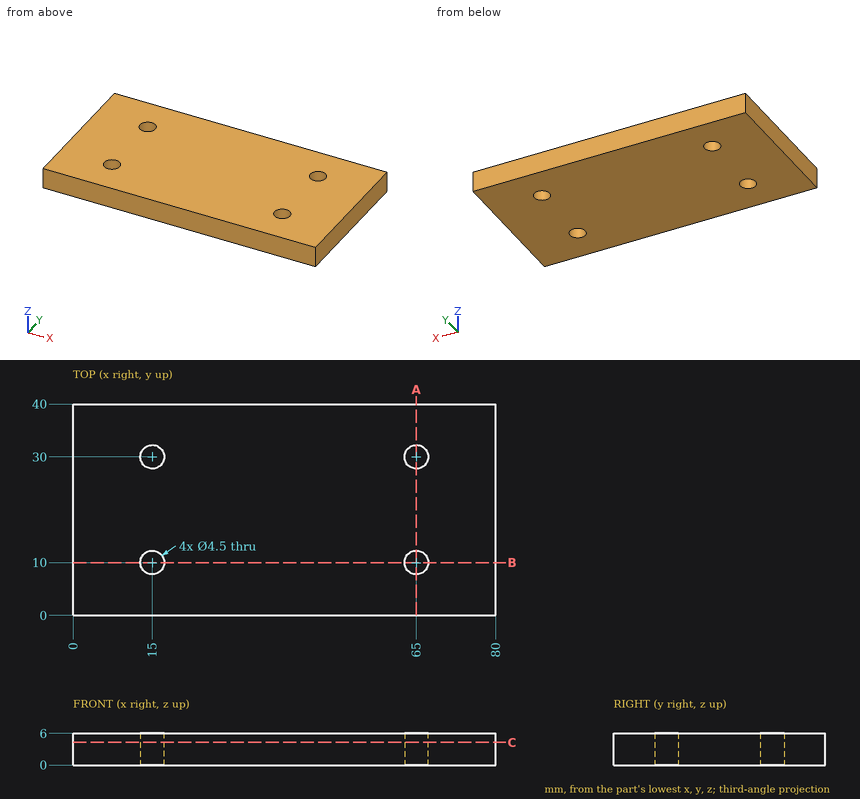
Drawing for the job (mm, zero at the part's lowest x, y, z). Coordinates: 2 decimals unless noted, no trailing zeros. Loops run counter-clockwise (first coordinate to the right, second up) from the corner with the lowest first, then second, coordinate; pieces in that order, holes last. Notation, with made-up numbers: (6, 50.5) - (51, 50.5) arc R14 cw to (51, 61.5) - close; hole circle Ø7 at (-10, 35.25). An arc over 180 degrees is marked (long way). Return JSON: item names as keys, results as strings.
1. Probe L1, parallel to Y at x = 65, z = 4; L2, parallel to X at y = 10, z = 3.65; L3, parallel to X at y = 29, z = 0.5. List the from-to ranges inside material, lowest first. Write a range as from..to.
Result:
{"L1": "y = 0..7.75, 12.25..27.75, 32.25..40", "L2": "x = 0..12.75, 17.25..62.75, 67.25..80", "L3": "x = 0..12.98, 17.02..62.98, 67.02..80"}
2. Band-saw the part on C-C (z = 4.3). Give the cut face in (x, y), and give its area (3 significant figures).
Result:
{"outline": "(0, 0) - (80, 0) - (80, 40) - (0, 40) - close; hole circle Ø4.5 at (15, 10); hole circle Ø4.5 at (15, 30); hole circle Ø4.5 at (65, 10); hole circle Ø4.5 at (65, 30)", "area": "3,140 mm2"}
3. Band-saw the part on B-B (y = 10). Give the cut face in (x, z), and give its area (3 significant figures).
Result:
{"outline": "(0, 0) - (12.75, 0) - (12.75, 6) - (0, 6) - close; (17.25, 0) - (62.75, 0) - (62.75, 6) - (17.25, 6) - close; (67.25, 0) - (80, 0) - (80, 6) - (67.25, 6) - close", "area": "426 mm2"}
4. Band-saw the part on A-A (x = 65). Give the cut face in (y, z), and give its area (3 significant figures).
Result:
{"outline": "(0, 0) - (7.75, 0) - (7.75, 6) - (0, 6) - close; (12.25, 0) - (27.75, 0) - (27.75, 6) - (12.25, 6) - close; (32.25, 0) - (40, 0) - (40, 6) - (32.25, 6) - close", "area": "186 mm2"}
